from build123d import *

# Parameters (mm, degrees)
EXTRUDE_1_DEPTH             = 30
SKETCH_2_W                  = 90
SKETCH_2_H                  = 20
CUT_EXTRUDE_1_DEPTH         = 61
SKETCH_3_W                  = 42.4
SKETCH_3_H                  = 42.4
CUT_EXTRUDE_2_DEPTH         = 7
SKETCH_4_W                  = 2.5
SKETCH_4_H                  = 3
SKETCH_5_W                  = 2.5
SKETCH_5_H                  = 3
HOLE_WIZARD_24_0_24_1_D     = 24
HOLE_WIZARD_24_0_24_1_DEPTH = 3
HOLE_WIZARD_3_2_3_2_1_D     = 3.2
HOLE_WIZARD_3_2_3_2_1_DEPTH = 3
HOLE_WIZARD_2_8_2_8_1_D     = 2.8
HOLE_WIZARD_2_8_2_8_1_DEPTH = 13
HOLE_WIZARD_3_2_3_2_2_D     = 3.2
HOLE_WIZARD_3_2_3_2_2_DEPTH = 10
HOLE_WIZARD_2_8_2_8_2_D     = 2.8
HOLE_WIZARD_2_8_2_8_2_DEPTH = 8.8
HOLE_WIZARD_2_8_2_8_3_D     = 2.8
HOLE_WIZARD_2_8_2_8_3_DEPTH = 8.8
EXTRUDE_2_DEPTH             = 10


with BuildPart() as part:
    # 草图1 → 凸台-拉伸1 (new body)
    with BuildSketch(Plane(origin=(0, 30, 0), x_dir=(1, 0, 0), z_dir=(0, 1, 0))):
        Polygon((-53.759164819, 38.577872891), (-53.759164819, -61.422127109), (-35.759164819, -79.767511878), (-37.57901599, -74.767511878), (-21.939313647, -74.767511878), (-23.759164819, -79.767511878), (6.240835181, -61.422127109), (6.240835181, 38.577872891), align=None)
    extrude(amount=-EXTRUDE_1_DEPTH)

    # 草图2 → 切除-拉伸1 (cut, through all)
    with BuildSketch(Plane.ZY.offset(53.759164819)):
        with Locations((6.422127109, 20)):
            Rectangle(SKETCH_2_W, SKETCH_2_H)
    extrude(amount=-CUT_EXTRUDE_1_DEPTH, mode=Mode.SUBTRACT)

    # 草图3 → 切除-拉伸2 (cut)
    with BuildSketch(Plane(origin=(0, 10, 0), x_dir=(-1, 0, 0), z_dir=(0, 1, 0))):
        with Locations((23.759164819, 7.622127109)):
            Rectangle(SKETCH_3_W, SKETCH_3_H)
    extrude(amount=-CUT_EXTRUDE_2_DEPTH, mode=Mode.SUBTRACT)

    # 草图4 → 旋转1 (revolve)
    with BuildSketch(Plane.XY.offset(-33.577872891)):
        with Locations((-44.509164819, 11.5)):
            Rectangle(SKETCH_4_W, SKETCH_4_H)
    revolve(axis=Axis((-45.759164819, 13, -33.577872891), (0, -1, 0)))

    # 草图5 → 旋转2 (revolve)
    with BuildSketch(Plane.XY.offset(-33.577872891)):
        with Locations((-0.509164819, 11.5)):
            Rectangle(SKETCH_5_W, SKETCH_5_H)
    revolve(axis=Axis((-1.759164819, 13, -33.577872891), (0, -1, 0)))

    # Ø24.0 (24) 直径孔1
    with Locations(Plane(origin=(0, 3, 0), x_dir=(1, 0, 0), z_dir=(0, 1, 0))):
        with Locations((-23.759164819, -7.622127109)):
            Hole(HOLE_WIZARD_24_0_24_1_D / 2, depth=HOLE_WIZARD_24_0_24_1_DEPTH)

    # Ø3.2 (3.2) 直径孔1
    with Locations(Plane(origin=(0, 3, 0), x_dir=(1, 0, 0), z_dir=(0, 1, 0))):
        with Locations((-8.259164819, -23.122127109), (-39.259164819, 7.877872891), (-8.259164819, 7.877872891), (-39.259164819, -23.122127109)):
            Hole(HOLE_WIZARD_3_2_3_2_1_D / 2, depth=HOLE_WIZARD_3_2_3_2_1_DEPTH)

    # Ø2.8 (2.8) 直径孔1
    with Locations(Plane(origin=(0, 13, 0), x_dir=(1, 0, 0), z_dir=(0, 1, 0))):
        with Locations((-45.759164819, 33.577872891), (-1.759164819, 33.577872891)):
            Hole(HOLE_WIZARD_2_8_2_8_1_D / 2, depth=HOLE_WIZARD_2_8_2_8_1_DEPTH)

    # Ø3.2 (3.2) 直径孔2
    with Locations(Plane(origin=(0, 10, 0), x_dir=(1, 0, 0), z_dir=(0, 1, 0))):
        with Locations((-45.759164819, -40.922127109), (-1.759164819, -40.922127109)):
            Hole(HOLE_WIZARD_3_2_3_2_2_D / 2, depth=HOLE_WIZARD_3_2_3_2_2_DEPTH)

    # Ø2.8 (2.8) 直径孔2
    with Locations(Plane.ZY.offset(53.759164819)):
        with Locations((-8.377872891, 5), (23.622127109, 5)):
            Hole(HOLE_WIZARD_2_8_2_8_2_D / 2, depth=HOLE_WIZARD_2_8_2_8_2_DEPTH)

    # Ø2.8 (2.8) 直径孔3
    with Locations(Plane.ZY.offset(2.559164819)):
        with Locations((-8.377872891, 5), (23.622127109, 5)):
            Hole(HOLE_WIZARD_2_8_2_8_3_D / 2, depth=HOLE_WIZARD_2_8_2_8_3_DEPTH)

    # 草图18 → 凸台-拉伸2 (add)
    with BuildSketch(Plane.XZ):
        Polygon((-35.759164819, 79.767511878), (-37.57901599, 74.767511878), (-21.939313647, 74.767511878), (-23.759164819, 79.767511878), align=None)
    extrude(amount=-EXTRUDE_2_DEPTH)


solid = part.part
Part model, mm, in its own coordinate system. A direction names the side the tool comes from. Give positions to 0.01 mm unless a question says otherwise; leave off trailing zeros. Loops run counter-clockwise (first coordinate to the right, second up) from the corner with the lowest first, then second, coordinate; pieces in that order, holes last.
(1) Drill centre lines: line 1 along X through (y, z) = (7.5, 4.5); line 2 along Y through (x, z) = (-45, 23.5); line 3 along Z through (x, y) = (-46, 9.25). Where is each one in solid material? Low to high.
Return value:
line 1: x = -53.76 to -44.96, -2.56 to 6.24
line 2: y = 0 to 3.61, 6.39 to 10
line 3: z = -38.58 to -34.96, -32.2 to 39.34, 42.5 to 69.33
(2) 3-axis set-ups, long thin cutter, end or side, ignore diameter. For faces 4 (the cylindrical face through (-37.66, 1.48, -7.95)), 5 (the flat face through (-23, 7, -13.578)): which of +Z, -Z, +X, -X, +Y, -Y reach the whole face in a straight line?
Return value:
face 4: +Y, -Y
face 5: +Y
(3) Band-saw the part on A-A (y = 5). Count the separate pieces of the cut face and the enclosed holes in it, and give its area (3 significant figures).
Return value:
separate pieces: 4
enclosed holes: 4
area: 4,740 mm2
(4) Band-saw the part on D-D (y = 18.25). Write the cut outline in (x, z).
Return value:
outline: (-53.76, 51.42) - (6.24, 51.42) - (6.24, 61.42) - (-23.76, 79.77) - (-21.94, 74.77) - (-37.58, 74.77) - (-35.76, 79.77) - (-53.76, 61.42) - close
(5) Band-saw the part on B-B (x = -32). Write the cut outline in (y, z) (3 decimals).
Return value:
outline: (0, -38.578) - (10, -38.578) - (10, -13.578) - (3, -13.578) - (3, -1.101) - (0, -1.101) - close; (0, 16.345) - (3, 16.345) - (3, 28.822) - (10, 28.822) - (10, 51.422) - (30, 51.422) - (30, 74.768) - (10, 74.768) - (10, 79.768) - (0, 79.768) - close
(6) Pin check, flat tips, straight feed: pin 1 (1.5 mm diameter, centred on x = -9, z = -25.5, fed in from +Y); pin 2 (10 mm diameter, centred on x = -39.5, y = 21.5, fed in from -Z); pin 3 (21 mm diameter, centred on x = -24.5, z = 9.5, fed in from +Y). Stop position of each tip, or through.
Return value:
pin 1: stops at y = 10
pin 2: stops at z = 51.42
pin 3: stops at y = 3
(7) Band-saw the part on C-C (z = 18.5). Write the cut outline in (x, y).
Return value:
outline: (-53.76, 0) - (-28.83, 0) - (-28.83, 3) - (-44.96, 3) - (-44.96, 10) - (-53.76, 10) - close; (-18.69, 0) - (6.24, 0) - (6.24, 10) - (-2.56, 10) - (-2.56, 3) - (-18.69, 3) - close
(8) Pull direction Z, two halves, no side cores. Call faces 1 (the flat face through (-47, 13, -35)), 2 (the flat face through (-23, 5, -38.578)), 3 (the flat face through (-23, 7, 28.822)): pulls with the +Z half, pulls with the -Z half, needs draft (parallel to the pull), parting line crosses it, or undercut.
Return value:
face 1: needs draft
face 2: pulls with the -Z half
face 3: undercut
